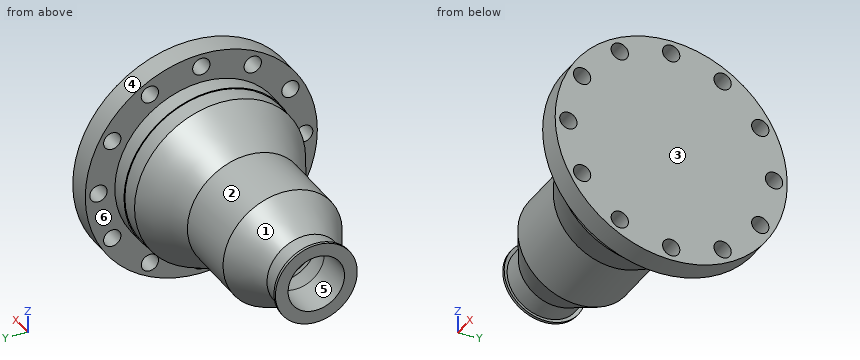
```python
from build123d import *

# Parameters (mm, degrees)
SKETCH_3_R           = 9.5
CUT_EXTRUDE_1_DEPTH  = 321.526909947
SKETCH_4_R           = 9.5
CUT_EXTRUDE_2_DEPTH  = 321.526909947
SKETCH_5_R           = 9.5
CUT_EXTRUDE_3_DEPTH  = 321.526909947
SKETCH_6_R           = 9.5
CUT_EXTRUDE_4_DEPTH  = 321.526909947
SKETCH_7_R           = 9.5
CUT_EXTRUDE_5_DEPTH  = 321.526909947
SKETCH_8_R           = 9.5
CUT_EXTRUDE_6_DEPTH  = 321.526909947
SKETCH_9_R           = 9.5
CUT_EXTRUDE_7_DEPTH  = 321.526909947
SKETCH_10_R          = 9.5
CUT_EXTRUDE_8_DEPTH  = 321.526909947
SKETCH_11_R          = 9.5
CUT_EXTRUDE_9_DEPTH  = 321.526909947
SKETCH_12_R          = 9.5
CUT_EXTRUDE_10_DEPTH = 321.526909947
SKETCH_13_R          = 9.5
CUT_EXTRUDE_11_DEPTH = 321.526909947
SKETCH_14_R          = 9.5
CUT_EXTRUDE_12_DEPTH = 321.526909947


with BuildPart() as part:
    # Эскиз1 → Повернуть1 (revolve)
    with BuildSketch(Plane.XY, mode=Mode.PRIVATE) as revolve_1_sk:
        Polygon((0, 0), (265, 0), (265, 127.5), (239, 127.5), (239, 100), (239, 95), (220, 95), (220, 94), (200, 94), (144, 65.5), (70, 65.5), (25, 41), (1.5, 41), (3, 45), (0, 45), align=None)
    revolve(revolve_1_sk.sketch.rotate(Axis((0, 0, 0), (1, 0, 0)), 90), axis=Axis((0, 0, 0), (1, 0, 0)))

    # Эскиз2 → Вырез-Повернуть1 (revolve, cut)
    with BuildSketch(Plane.XY, mode=Mode.PRIVATE) as cut_revolve_1_sk:
        with BuildLine():
            Line((0, 0), (220, 0))
            Line((220, 0), (220, 38.502577))
            Line((220, 38.502577), (200, 38.502577))
            Line((200, 38.502577), (200, 55))
            Line((200, 55), (147.669872, 55))
            ThreePointArc((147.669872, 55), (146.273624348, 54.108499061), (146.669872, 52.5))
            Line((146.669872, 52.5), (143.5, 52.5))
            ThreePointArc((143.5, 52.5), (142.75, 52.602347572), (142, 52.5))
            Line((142, 52.5), (90, 52.5))
            ThreePointArc((90, 52.5), (79.13262933, 46.740617582), (70, 38.502577))
            Line((70, 38.502577), (42, 31))
            Line((42, 31), (0, 31))
            Line((0, 31), (0, 0))
        make_face()
    revolve(cut_revolve_1_sk.sketch.rotate(Axis((0, 0, 0), (1, 0, 0)), 90), axis=Axis((0, 0, 0), (1, 0, 0)), mode=Mode.SUBTRACT)

    # Эскиз3 → Вырез-Вытянуть1 (cut, through all)
    with BuildSketch(Plane(origin=(0, 0, 0), x_dir=(0, 0, -1), z_dir=(1, 0, 0))):
        with Locations((0, 113)):
            Circle(SKETCH_3_R)
    extrude(amount=CUT_EXTRUDE_1_DEPTH, mode=Mode.SUBTRACT)

    # Эскиз4 → Вырез-Вытянуть2 (cut, through all)
    with BuildSketch(Plane(origin=(0, 0, 0), x_dir=(0, 0, -1), z_dir=(1, 0, 0))):
        with Locations((-56.5, 97.860870628)):
            Circle(SKETCH_4_R)
    extrude(amount=CUT_EXTRUDE_2_DEPTH, mode=Mode.SUBTRACT)

    # Эскиз5 → Вырез-Вытянуть3 (cut, through all)
    with BuildSketch(Plane(origin=(0, 0, 0), x_dir=(0, 0, -1), z_dir=(1, 0, 0))):
        with Locations((-97.860870628, 56.5)):
            Circle(SKETCH_5_R)
    extrude(amount=CUT_EXTRUDE_3_DEPTH, mode=Mode.SUBTRACT)

    # Эскиз6 → Вырез-Вытянуть4 (cut, through all)
    with BuildSketch(Plane(origin=(0, 0, 0), x_dir=(0, 0, -1), z_dir=(1, 0, 0))):
        with Locations((-113, 0)):
            Circle(SKETCH_6_R)
    extrude(amount=CUT_EXTRUDE_4_DEPTH, mode=Mode.SUBTRACT)

    # Эскиз7 → Вырез-Вытянуть5 (cut, through all)
    with BuildSketch(Plane(origin=(0, 0, 0), x_dir=(0, 0, -1), z_dir=(1, 0, 0))):
        with Locations((-97.860870628, -56.5)):
            Circle(SKETCH_7_R)
    extrude(amount=CUT_EXTRUDE_5_DEPTH, mode=Mode.SUBTRACT)

    # Эскиз8 → Вырез-Вытянуть6 (cut, through all)
    with BuildSketch(Plane(origin=(0, 0, 0), x_dir=(0, 0, -1), z_dir=(1, 0, 0))):
        with Locations((-56.5, -97.860870628)):
            Circle(SKETCH_8_R)
    extrude(amount=CUT_EXTRUDE_6_DEPTH, mode=Mode.SUBTRACT)

    # Эскиз9 → Вырез-Вытянуть7 (cut, through all)
    with BuildSketch(Plane(origin=(0, 0, 0), x_dir=(0, 0, -1), z_dir=(1, 0, 0))):
        with Locations((0, -113)):
            Circle(SKETCH_9_R)
    extrude(amount=CUT_EXTRUDE_7_DEPTH, mode=Mode.SUBTRACT)

    # Эскиз10 → Вырез-Вытянуть8 (cut, through all)
    with BuildSketch(Plane(origin=(0, 0, 0), x_dir=(0, 0, -1), z_dir=(1, 0, 0))):
        with Locations((56.5, -97.860870628)):
            Circle(SKETCH_10_R)
    extrude(amount=CUT_EXTRUDE_8_DEPTH, mode=Mode.SUBTRACT)

    # Эскиз11 → Вырез-Вытянуть9 (cut, through all)
    with BuildSketch(Plane(origin=(0, 0, 0), x_dir=(0, 0, -1), z_dir=(1, 0, 0))):
        with Locations((97.860870628, -56.5)):
            Circle(SKETCH_11_R)
    extrude(amount=CUT_EXTRUDE_9_DEPTH, mode=Mode.SUBTRACT)

    # Эскиз12 → Вырез-Вытянуть10 (cut, through all)
    with BuildSketch(Plane(origin=(0, 0, 0), x_dir=(0, 0, -1), z_dir=(1, 0, 0))):
        with Locations((113, 0)):
            Circle(SKETCH_12_R)
    extrude(amount=CUT_EXTRUDE_10_DEPTH, mode=Mode.SUBTRACT)

    # Эскиз13 → Вырез-Вытянуть11 (cut, through all)
    with BuildSketch(Plane(origin=(0, 0, 0), x_dir=(0, 0, -1), z_dir=(1, 0, 0))):
        with Locations((97.860870628, 56.5)):
            Circle(SKETCH_13_R)
    extrude(amount=CUT_EXTRUDE_11_DEPTH, mode=Mode.SUBTRACT)

    # Эскиз14 → Вырез-Вытянуть12 (cut, through all)
    with BuildSketch(Plane(origin=(0, 0, 0), x_dir=(0, 0, -1), z_dir=(1, 0, 0))):
        with Locations((56.5, 97.860870628)):
            Circle(SKETCH_14_R)
    extrude(amount=CUT_EXTRUDE_12_DEPTH, mode=Mode.SUBTRACT)


solid = part.part
```
CAD build for the part. Positions are in the model's coordinates, mm. Face numbers are marked on the shaded views. A direction names the side the tool comes from. Coordinates: 2 decimals unless noted, no trailing zeros. Order: outer loops, then holes, each group sorted by start corner. A loop starts at its lowest first (then second) coordinate and runs counter-clockwise, first axis right, second up. Notation, with made-up numbers: M -10.5,37 L 3.5,37 A23 cw 3.5,67 Z; hole C 27,16 d8. An arc over 180 degrees is marked long. Answer as CSV lines item,"result".
1) 3-axis set-ups, long thin cutter, end or side, ignore diameter. For the marked faces 1, 2 and 3: which of +Z, -Z, +X, -X, +Y, -Y reach the whole face in a straight line?
Verdict:
face 1,"none"
face 2,"-X"
face 3,"+Z, -Z, +X, +Y, -Y"
2) Cut at A-A (z = 113). List the corners of the cut face in (x, y).
Verdict:
outline,"M 239,-59.05 L 265,-59.05 L 265,-9.5 L 239,-9.5 Z; M 239,9.5 L 265,9.5 L 265,59.05 L 239,59.05 Z"
3) Cut at B-B (x = 106). List the corners of the cut face in (y, z).
Verdict:
outline,"C 0,0 d131; hole C 0,0 d105"
4) Drill centre lines: L1, parallel to Y at x = 257.75, z = 0; L2, parallel to Y at x = 258, z = -56; L3, parallel to Y at x = 215.25, z = 0. Where is each one in solid material? Low to high. Write a range as from..to.
Verdict:
L1,"-127.5..-122.5, -103.5..103.5, 122.5..127.5"
L2,"-114.54..-107.35, -88.37..88.37, 107.35..114.54"
L3,"-94..-38.5, 38.5..94"
5) Cut at C-C (y = 0). Give the number of separate pieces and of enclosed holes in the cut face, then the cut area to 3 significant figures.
Verdict:
separate pieces,"3"
enclosed holes,"0"
area,"18,700 mm2"
6) Flat gauge pins, fed straight in: P1, Ø15, axis at y = -56.5, z = 97.86, coming from the +X side; P2, Ø3, axis at x = 61, z = -53, coming from the +Y side; P3, Ø1, axis at y = 80, z = -14, coming from the -X side; P4, Ø2, axis at x = 172.5, z = -39.5, coming from the -Y side. Where does each tip first touch, or does it go through?
Verdict:
P1,"through"
P2,"y = 32.39"
P3,"x = 173.9"
P4,"y = -70.38"
7) Mould opens along Z. For the marked faces 4, 5 and 6 say: released by +Z, released by -Z, zero draft, split by the parting line, or undercut.
Verdict:
face 4,"split by the parting line"
face 5,"undercut"
face 6,"zero draft"
